from build123d import *

# Parameters (mm, degrees)
SKETCH1_R                 = 12.5
BOSS_EXTRUDE1_DEPTH       = 16
BOSS_EXTRUDE2_DEPTH       = 8
SKETCH1_6_R               = 8
BOSS_EXTRUDE3_DEPTH       = 80
BOSS_EXTRUDE4_START       = -24
SKETCH1_7_W               = 8
SKETCH1_7_H               = 32
BOSS_EXTRUDE4_DEPTH       = 32
FILLET1_RADIUS            = 16
FILLET1_LENGTH            = 8
F_8_0MM_DOWEL_HOLE1_D     = 8
F_8_0MM_DOWEL_HOLE1_DEPTH = 8
BOSS_EXTRUDE5_REACH       = 169.236
SKETCH3_R                 = 4
FILLET2_R                 = 10


with BuildPart() as part:
    # Sketch1 → Boss-Extrude1 (new body)
    with BuildSketch(Plane.XY):
        with BuildLine():
            Line((80, 8), (80, 0))
            Line((80, 0), (108, 0))
            ThreePointArc((108, 0), (128, 20), (108, 40))
            ThreePointArc((108, 40), (99.076043738, 37.898687232), (92.027289799, 32.036300463))
            Line((92.027289799, 32.036300463), (73.914638236, 8))
            Line((73.914638236, 8), (80, 8))
        make_face()
        with Locations((108, 20)):
            Circle(SKETCH1_R, mode=Mode.SUBTRACT)
    boss_extrude1 = extrude(amount=-BOSS_EXTRUDE1_DEPTH)

    # Sketch1<5> → Boss-Extrude2 (add)
    with BuildSketch(Plane.XY):
        with BuildLine():
            Line((9, 40), (9, 8))
            Line((9, 8), (73.914638236, 8))
            Line((73.914638236, 8), (92.027289799, 32.036300463))
            ThreePointArc((92.027289799, 32.036300463), (99.076043738, 37.898687232), (108, 40))
            Line((108, 40), (9, 40))
        make_face()
    boss_extrude2 = extrude(amount=-BOSS_EXTRUDE2_DEPTH)

    # Sketch1<6> → Boss-Extrude3 (add)
    # profile 1 of 3: a face of its own
    with BuildSketch(Plane.XY):
        Polygon((9, 8), (9, 0), (0, 0), (0, 40), (9, 40), align=None)
    # profile 2 of 3: a face of its own
    with BuildSketch(Plane.XY):
        Polygon((9, 8), (9, 0), (48, 0), (80, 0), (80, 8), (73.914638236, 8), align=None)
    # profile 3 of 3: a face of its own
    with BuildSketch(Plane.XY):
        with BuildLine():
            Line((80, 0), (48, 0))
            Line((48, 0), (48, -16))
            ThreePointArc((48, -16), (64, -32), (80, -16))
            Line((80, -16), (80, 0))
        make_face()
        with Locations((64, -16)):
            Circle(SKETCH1_6_R, mode=Mode.SUBTRACT)
    extrude(amount=-BOSS_EXTRUDE3_DEPTH)

    # Mirror1: Boss-Extrude1, Boss-Extrude2 across plane
    add(boss_extrude1.mirror(Plane.XY.offset(-40)))
    add(boss_extrude2.mirror(Plane.XY.offset(-40)))

    # Sketch1<7> → Boss-Extrude4 (add)
    with BuildSketch(Plane.XY.offset(BOSS_EXTRUDE4_START)):
        with Locations((-4, 16)):
            Rectangle(SKETCH1_7_W, SKETCH1_7_H)
    extrude(amount=-BOSS_EXTRUDE4_DEPTH)

    # Fillet1: full round fillet: the end face becomes a half cylinder, R = half its width
    fillet1_face = Plane((-4, 32, -40), x_dir=(-1, 0, 0), z_dir=(0, 1, 0))  # on the end face: x along it, z out of the body
    fillet1_slab = fillet1_face.offset(-FILLET1_RADIUS / 2) * Box(FILLET1_LENGTH, 2 * FILLET1_RADIUS, FILLET1_RADIUS, mode=Mode.PRIVATE)  # the body's end, R deep
    fillet1_round = Plane((-4, 16, -40), x_dir=(0, 1, 0), z_dir=(-1, 0, 0)) * Cylinder(FILLET1_RADIUS, FILLET1_LENGTH, mode=Mode.PRIVATE)  # its axis R under the face
    add(fillet1_slab - fillet1_round, mode=Mode.SUBTRACT)

    # Ø8.0mm Dowel Hole1
    with Locations(Plane(origin=(-8, 16, -40), x_dir=(0, -1, 0), z_dir=(-1, 0, 0))):
        with Locations((0, 0)):
            Hole(F_8_0MM_DOWEL_HOLE1_D / 2, depth=F_8_0MM_DOWEL_HOLE1_DEPTH)

    # Sketch3 → Boss-Extrude5 (add, up to next)
    with BuildSketch(Plane(origin=(0, 40, 0), x_dir=(1, 0, 0), z_dir=(0, 1, 0)), mode=Mode.PRIVATE) as boss_extrude5_sk1:
        with BuildLine():
            Line((32, 72), (9, 72))
            Line((9, 72), (9, 48.031280577))
            ThreePointArc((9, 48.031280577), (11.169048105, 53.508506152), (16.5, 56.015640289))
            ThreePointArc((16.5, 56.015640289), (21.830951895, 58.522774425), (24, 64))
            ThreePointArc((24, 64), (26.343145751, 69.656854249), (32, 72))
        make_face()
        with Locations(Location((16, 64, 0), (0, 0, 270))):
            Circle(SKETCH3_R, mode=Mode.SUBTRACT)
    boss_extrude5_tool1 = extrude(boss_extrude5_sk1.sketch, amount=-BOSS_EXTRUDE5_REACH, mode=Mode.PRIVATE) - part.part
    # Sketch3 → Boss-Extrude5 (add, up to next)
    with BuildSketch(Plane(origin=(0, 40, 0), x_dir=(1, 0, 0), z_dir=(0, 1, 0)), mode=Mode.PRIVATE) as boss_extrude5_sk2:
        with BuildLine():
            ThreePointArc((16.5, 23.984359711), (11.169048105, 26.491493848), (9, 31.968719423))
            Line((9, 31.968719423), (9, 8))
            Line((9, 8), (32, 8))
            ThreePointArc((32, 8), (26.343145751, 10.343145751), (24, 16))
            ThreePointArc((24, 16), (21.830951895, 21.477225575), (16.5, 23.984359711))
        make_face()
        with Locations(Location((16, 16, 0), (0, 0, 270))):
            Circle(SKETCH3_R, mode=Mode.SUBTRACT)
    boss_extrude5_tool2 = extrude(boss_extrude5_sk2.sketch, amount=-BOSS_EXTRUDE5_REACH, mode=Mode.PRIVATE) - part.part
    add(boss_extrude5_tool1.solids().sort_by_distance((20.5, 40, -71.66781))[0])
    add(boss_extrude5_tool2.solids().sort_by_distance((10.926925, 40, -26.264059))[0])

    # Fillet2
    fillet2_edges = [part.edges().sort_by_distance(p)[0] for p in [
        (0, 20, 0),
        (0, 20, -80),
    ]]
    fillet(fillet2_edges, radius=FILLET2_R)


solid = part.part
Here's how the part is built. I have some questions about the finished solid (model axes, mm). A direction names the side the tool comes from. Give positions to 0.01 mm unless a question says otherwise; leave off trailing zeros. Order: outer loops, then holes, each group sorted by start corner. A loop starts at its lowest first (then second) coordinate and runs counter-clockwise, first axis right, second up. Notation, with made-up numbers: (32, 20.25) -> (62, 20.25) arc R21 cw to (62, 27.25) -> close; hole circle Ø9 at (10, 10). An arc over 180 degrees is marked (long way). Use a Markdown table: item, result. Add a question column.
Item 1: Imagine slicing it at B-B on y = -10.5. Please give me the cut outline in (x, z), plus the area to 3 significant figures.
Item 2: Imagine slicing it at C-C on z = -42. Please give me the cut outline in (x, y).
Item 3: Imagine slicing it at D-D on x = 100. Please give me the cut outline in (y, z), plus the area to 3 significant figures.
Item 4: Imagine slicing it at A-A on x = 64. Please give me the cut outline in (y, z), plus the area to 3 significant figures.
Item 5: For faces 1 (the face through (94, 0, -72)), 2 (the face through (9, 24, -40)), 3 (the face through (61, 24, -72)), which set-ups out of +Z, -Z, +X, -X, +Y, -Y let a thin tool reach every point of the face, with its end or its side?
Item 6: If we mould it in two halves opening along Y, with no side actions, what happens to faces 4 (the face through (119.547, 15.212, -7.888)), 5 (the face through (20, 0, -39)), 6 (the face through (16, 8, -16)), 7 (the face through (48, -8, -39))? For each: pulls with the +Y half, pulls with the -Y half, needs draft (parallel to the pull), parting line crosses it, or undercut.
Item 7: I need wall thicknesses on line 1 (Z direction, x = 40, y = 15.5); line 2 (Y direction, x = 64, z = -53); line 3 (Y direction, x = 108, z = -12.5). Which ranges of each line are inside material? Lowest first, please.
Item 8: Will these pins go through, and if not, where does the flat tip stop? pin 1 (8 mm diameter, centred on x = 89, z = -6.5, fed in from -Y); pin 2 (8 mm diameter, centred on y = 9, z = -23.5, fed in from +X); pin 3 (2.5 mm diameter, centred on y = 17, z = -40, fed in from -X).
Data:
| question | item | result |
|---|---|---|
| 1 | outline | (48, -80) -> (58.19, -80) -> (58.19, 0) -> (48, 0) -> close; (69.81, -80) -> (80, -80) -> (80, 0) -> (69.81, 0) -> close |
| 1 | area | 1,630 mm² |
| 2 | outline | (-8, 0) -> (48, 0) -> (48, -16) arc R16 ccw to (80, -16) -> (80, 8) -> (9, 8) -> (9, 40) -> (0, 40) -> (0, 31.87) -> (-8, 31.87) -> (-8, 19.46) -> (0, 19.46) -> (0, 12.54) -> (-8, 12.54) -> close; hole circle Ø16 at (64, -16) |
| 3 | outline | (0, -80) -> (10.4, -80) -> (10.4, -64) -> (0, -64) -> close; (0, -16) -> (10.4, -16) -> (10.4, 0) -> (0, 0) -> close; (29.6, -80) -> (40, -80) -> (40, -72) -> (38.33, -72) -> (38.33, -64) -> (29.6, -64) -> close; (29.6, -16) -> (38.33, -16) -> (38.33, -8) -> (40, -8) -> (40, 0) -> (29.6, 0) -> close |
| 3 | area | 639 mm² |
| 4 | outline | (-32, -80) -> (-24, -80) -> (-24, 0) -> (-32, 0) -> close; (-8, -80) -> (40, -80) -> (40, -72) -> (8, -72) -> (8, -8) -> (40, -8) -> (40, 0) -> (-8, 0) -> close |
| 4 | area | 2,430 mm² |
| 5 | face 1 | +Z, -Z, +X, -Y |
| 5 | face 2 | +X, +Y |
| 5 | face 3 | +Y |
| 6 | face 4 | undercut |
| 6 | face 5 | pulls with the -Y half |
| 6 | face 6 | pulls with the +Y half |
| 6 | face 7 | needs draft |
| 7 | line 1 | z = -80 to -72, -8 to 0 |
| 7 | line 2 | y = -32 to -24, -8 to 8 |
| 7 | line 3 | y = 0 to 7.5, 32.5 to 40 |
| 8 | pin 1 | stops at y = 0 |
| 8 | pin 2 | stops at x = 80 |
| 8 | pin 3 | stops at x = 0 |
